```python
from build123d import *

# Parameters (mm, degrees)
CROQUIS1_W              = 28
CROQUIS1_H              = 4.1
CROQUIS3_W              = 12
CROQUIS3_H              = 13
SALIENTE_EXTRUIR1_DEPTH = 1
CROQUIS4_W              = 12
CROQUIS4_H              = 13
SALIENTE_EXTRUIR2_DEPTH = 1
REDONDEO1_R             = 0.5
CORTAR_EXTRUIR1_REACH   = 30
CROQUIS5_R              = 3.075


with BuildPart() as part:
    # Croquis1 → Revolución1 (revolve)
    with BuildSketch(Plane.XY):
        with Locations((0, 2.05)):
            Rectangle(CROQUIS1_W, CROQUIS1_H)
    revolve(axis=Axis((-14, 0, 0), (1, 0, 0)))

    # Croquis3 → Saliente-Extruir1 (add)
    with BuildSketch(Plane(origin=(11.8, 0, 0), x_dir=(0, 0, -1), z_dir=(1, 0, 0))):
        Rectangle(CROQUIS3_W, CROQUIS3_H)
    extrude(amount=SALIENTE_EXTRUIR1_DEPTH)

    # Croquis4 → Saliente-Extruir2 (add)
    with BuildSketch(Plane.ZY.offset(14)):
        Rectangle(CROQUIS4_W, CROQUIS4_H)
    extrude(amount=-SALIENTE_EXTRUIR2_DEPTH)

    # Redondeo1
    redondeo1_edges = [part.edges().sort_by_distance(p)[0] for p in [
        (12.3, 6.5, 6),
        (12.3, -6.5, 6),
        (12.3, -6.5, -6),
        (12.3, 6.5, -6),
        (-13.5, -6.5, -6),
        (-13.5, 6.5, -6),
        (-13.5, 6.5, 6),
        (-13.5, -6.5, 6),
    ]]
    fillet(redondeo1_edges, radius=REDONDEO1_R)

    # Croquis5 → Cortar-Extruir1 (cut, up to next)
    with BuildSketch(Plane(origin=(14, 0, 0), x_dir=(0, 0, -1), z_dir=(1, 0, 0)), mode=Mode.PRIVATE) as cortar_extruir1_sk1:
        Circle(CROQUIS5_R)
    cortar_extruir1_tool1 = extrude(cortar_extruir1_sk1.sketch, amount=-CORTAR_EXTRUIR1_REACH, mode=Mode.PRIVATE) & part.part
    add(cortar_extruir1_tool1.solids().sort_by_distance((14, 0, 0))[0], mode=Mode.SUBTRACT)


solid = part.part
```
Can you work these out from the model? Positions are in its coordinate system, mm. A direction names the side the tool comes from. Give positions to 0.01 mm unless a question says otherwise; leave off trailing zeros. Loops run counter-clockwise (first coordinate to the right, second up) from the corner with the lowest first, then second, coordinate; pieces in that order, holes last. Notation, with made-up numbers: M 26.5,26.5 L 79.5,26.5 A25 ccw 79.5,51.5 Z; hole C 72,62.5 d8. An arc over 180 degrees is marked long. Answer in a Markdown table with one row per item.
1. Suppose I cut it at B-B on y = -1.25. Write out the boundary of the cut face in (x, z).
Taken from the geometry:
| item | result |
|---|---|
| outline | M -14,-6 L -13,-6 L -13,-3.9 L 11.8,-3.9 L 11.8,-6 L 12.8,-6 L 12.8,-3.9 L 14,-3.9 L 14,-2.81 L -14,-2.81 Z; M -14,2.81 L 14,2.81 L 14,3.9 L 12.8,3.9 L 12.8,6 L 11.8,6 L 11.8,3.9 L -13,3.9 L -13,6 L -14,6 Z |
2. Suppose I cut it at D-D on x = -5.75. Write out the boundary of the cut face in (y, z) (3 decimals).
Taken from the geometry:
| item | result |
|---|---|
| outline | C 0,0 d8.2; hole C 0,0 d6.15 |
3. Which directions (+Z, -Z, +X, -X, +Y, -Y) give clear straight access to the entire face, cutting with the end or side of a thin tool? Please do faces 5 (the flat face through (-13, 2, -4)), 6 (the cylindrical face through (13.408, -0.534, 4.065)), 7 (the flat face through (-13.5, -0.1, 6)).
Taken from the geometry:
| item | result |
|---|---|
| face 5 | none |
| face 6 | +X |
| face 7 | +Z, +X, -X, +Y, -Y |
4. Suppose I cut it at A-A on z = 0. Write out the boundary of the cut face in (x, y) (3 decimals).
Taken from the geometry:
| item | result |
|---|---|
| outline | M -14,-6.5 L -13,-6.5 L -13,-4.1 L 11.8,-4.1 L 11.8,-6.5 L 12.8,-6.5 L 12.8,-4.1 L 14,-4.1 L 14,-3.075 L -14,-3.075 Z; M -14,3.075 L 14,3.075 L 14,4.1 L 12.8,4.1 L 12.8,6.5 L 11.8,6.5 L 11.8,4.1 L -13,4.1 L -13,6.5 L -14,6.5 Z |
5. Thinking about a two-plate mould opening in X: for faces 1 (the flat face through (11.8, 2, 4)), 2 (the flat face through (14, 0.9, 3.1)), 3 (the flat face through (-14, 2, -3)), 4 (the flat face through (12, 0, -6)), which applies, released by +X, released by -X, zero draft, split by the parting line, or undercut?
Taken from the geometry:
| item | result |
|---|---|
| face 1 | undercut |
| face 2 | released by +X |
| face 3 | released by -X |
| face 4 | zero draft |
6. Suppose I cut it at C-C on y = 5.5. Write out the boundary of the cut face in (x, z), plus the area to 3 significant figures.
Taken from the geometry:
| item | result |
|---|---|
| outline | M -14,-6 L -13,-6 L -13,6 L -14,6 Z; M 11.8,-6 L 12.8,-6 L 12.8,6 L 11.8,6 Z |
| area | 24.0 mm² |
7. For pin 1 Ø2 at (x, y) = (-6.5, -0.5) entering from +Z; pin 2 Ø4 at (x, z) = (3, 4.5) entering from +Y; pin 3 Ø5 at (y, z) = (0, 0) entering from +X; pin 4 Ø3 at (x, z) = (7.5, -4) entering from -Y, each with a flat end and sliding along its axis, tell me the tip position at first contact or that it passes through.
Taken from the geometry:
| item | result |
|---|---|
| pin 1 | stops at z = 4.1 |
| pin 2 | stops at y = 3.25 |
| pin 3 | passes through |
| pin 4 | stops at y = -3.25 |
8. If I drill on line 1 along X through (y, z) = (0.5, -5); line 2 along Z through (x, y) = (-12, 0.5); line 3 along Y through (x, z) = (12.25, 2), over which ranges is the centre line in solid material (lowest first)?
Taken from the geometry:
| item | result |
|---|---|
| line 1 | x = -14 to -13, 11.8 to 12.8 |
| line 2 | z = -4.07 to -3.03, 3.03 to 4.07 |
| line 3 | y = -6.5 to -2.34, 2.34 to 6.5 |
